Solid Edge part; units mm, degrees
sketch "Sketch1" plane through (0, 0, 0) normal (0, -1, 0) x (1, 0, 0)
  arc A0 (-15, -5) -> (-15, 5) centre (-15, 0) cw
  line L0 (-15, 5) -> (15, 5)
  arc A1 (15, 5) -> (15, -5) centre (15, 0) cw
  line L1 (15, -5) -> (-15, -5)
  circle A2 centre (15, 0) radius 2.5
  circle A3 centre (-15, 0) radius 2.5
extrude "Protrusion1" add sketch "Sketch1" along normal mid plane 10
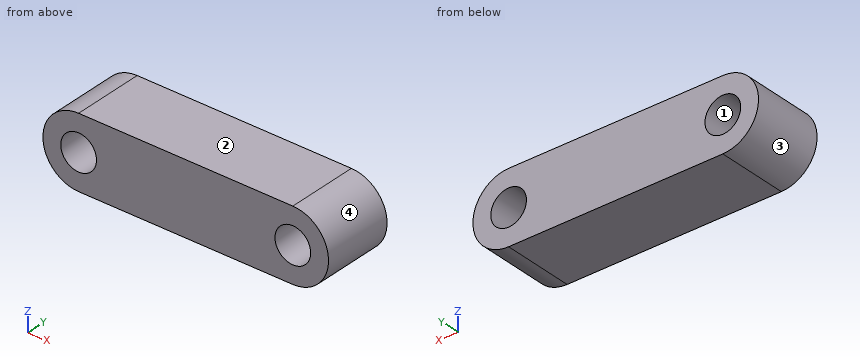
Geometry check sheet. Reference: the model listing, model coordinates, mm. Face numbers are marked on the shaded views. Coordinates: 2 decimals unless noted, no trailing zeros. Write each loop counter-clockwise with the first axis right and the second up, starting at its lowest first coordinate (ties: lowest second). Pieces come first, ordered by that corner, then holes. Notation, with made-up numbers: (29, 73.5) -> (81, 73.5) arc R27 ccw to (81, 89.5) -> close; hole circle Ø7 at (-33.75, 40). An arc over 180 degrees is marked (long way). Use CSV: the item, a comma, the result in double quotes. Start each with the question number.
Item 1: Thickness scan on line 1 (Z direction, x = -15, y = 1.5); line 2 (X direction, y = -3.5, z = 1); line 3 (X direction, y = -1.5, z = 2). Record the ranges inside material, lowest first.
Item 2: Cross-section at A-A, the plane z = 0. Record the cut outline in (x, y).
Item 3: Cross-section at C-C, the plane z = 4.25. Record the cut outline in (x, y), plus the area to 3 significant figures.
Item 4: Depth check by flat-ended pin: pin 1 Ø1.5 at (y, z) = (1.5, -1) entering from +X. Enter the tip coordinate at first touch or a pass-through.
Item 5: Cross-section at B-B, the plane y = -4.5. Record the cut outline in (x, z).
Item 6: Mould release check, pull along X, two halves, no side actions. Record for the marked faces 1, 2, 3 and 4: released by +X, released by -X, zero draft, split by the parting line, or undercut.
Answers:
1,line 1,"-5 to -2.5, 2.5 to 5"
1,line 2,"-19.9 to -17.29, -12.71 to 12.71, 17.29 to 19.9"
1,line 3,"-19.58 to -16.5, -13.5 to 13.5, 16.5 to 19.58"
2,outline,"(-20, -5) -> (-17.5, -5) -> (-17.5, 5) -> (-20, 5) -> close; (-12.5, -5) -> (12.5, -5) -> (12.5, 5) -> (-12.5, 5) -> close; (17.5, -5) -> (20, -5) -> (20, 5) -> (17.5, 5) -> close"
3,outline,"(-17.63, -5) -> (17.63, -5) -> (17.63, 5) -> (-17.63, 5) -> close"
3,area,"353 mm^2"
4,pin 1,"x = 19.99"
5,outline,"(-15, -5) -> (15, -5) arc R5 ccw to (15, 5) -> (-15, 5) arc R5 ccw to start; hole circle Ø5 at (-15, 0); hole circle Ø5 at (15, 0)"
6,face 1,"undercut"
6,face 2,"zero draft"
6,face 3,"released by -X"
6,face 4,"released by +X"
